Here's how the part is built. I have some questions about the finished solid (model axes, mm). A direction names the side the tool comes from. Coordinates: 2 decimals unless noted, no trailing zeros. Order: outer loops, then holes, each group sorted by start corner. A loop starts at its lowest first (then second) coordinate and runs counter-clockwise, first axis right, second up. Notation, with made-up numbers: (70, 28) -> (78, 28) arc R36 cw to (78, 63) -> close; hole circle Ø10 at (87.5, 17.5). An arc over 180 degrees is marked (long way). One line per item, written item: value. Start each with the question number.
```python
from build123d import *

# Parameters (mm, degrees)
SKETCH1_R           = 9.5
BOSS_EXTRUDE1_DEPTH = 1
SKETCH2_R           = 8.5
BOSS_EXTRUDE3_DEPTH = 4
SKETCH3_R           = 8.5
BOSS_EXTRUDE4_DEPTH = 4
CUT_EXTRUDE1_DEPTH  = 17.748134224


with BuildPart() as part:
    # Sketch1 → Boss-Extrude1 (new, symmetric)
    with BuildSketch(Plane.YZ):
        with Locations(Location((0, 0, 0), (0, 0, 270))):
            Circle(SKETCH1_R)
    extrude(amount=BOSS_EXTRUDE1_DEPTH, both=True)

    # Sketch2 → Boss-Extrude3 (add)
    with BuildSketch(Plane.YZ.offset(1)):
        with Locations(Location((-1, 0, 0), (0, 0, 180))):
            Circle(SKETCH2_R)
    extrude(amount=BOSS_EXTRUDE3_DEPTH)

    # Sketch3 → Boss-Extrude4 (add)
    with BuildSketch(Plane(origin=(-1, 0, 0), x_dir=(0, -1, 0), z_dir=(-1, 0, 0))):
        with Locations(Location((-1, 0, 0), (0, 0, 179.999143376))):
            Circle(SKETCH3_R)
    extrude(amount=BOSS_EXTRUDE4_DEPTH)

    # Sketch4 → Cut-Extrude1 (cut, through all)
    with BuildSketch(Plane.YZ.offset(5)):
        with BuildLine():
            Line((-1.5, 4.874423043), (-1.5, 6.7))
            Line((-1.5, 6.7), (1.5, 6.7))
            Line((1.5, 6.7), (1.5, 4.874423043))
            ThreePointArc((1.5, 4.874423043), (0, -5.1), (-1.5, 4.874423043))
        make_face()
    extrude(amount=-CUT_EXTRUDE1_DEPTH, mode=Mode.SUBTRACT)


solid = part.part
```
Q1. Imagine slicing it at A-A (x = 3). Write out the boundary of the cut face in (y, z), plus the area to 3 significant figures.
Q2. Imagine slicing it at D-D (z = -6.25). Write out the boundary of the cut face in (x, y).
Q3. Imagine slicing it at C-C (y = 0). Write out the boundary of the cut face in (x, z).
Q4. For P1, Ø2, axis at x = -2.5, y = 4.5, coming from the +Z side; P2, Ø0.5, axis at x = 2, z = 5.5, coming from the +Y side; P3, Ø1.5, axis at x = 2.5, z = 1.5, coming from the +Y side, each with a flat end and sliding along its axis, tell me the tip position at first contact or that it passes through.
Q5. For faces 4 (the face through (2.97, -9.11, -2.55)), 5 (the face through (-2.97, -0.84, 8.3)), 6 (the face through (0, 1.5, 6)), which set-ups out of +Z, -Z, +X, -X, +Y, -Y let a thin tool reach every point of the face, with its end or its side?
Q6. I need wall thicknesses on line 1 (Y direction, x = -1.25, z = 0); line 2 (Z direction, x = 0, y = 0); line 3 (Y direction, x = -0.5, z = 4). Which ranges of each line are inside material? Lowest first, please.
Q7. If we mould it in two halves opening along Z, with no side actions, what happens to faces 1 (the face through (0.01, -5.78, 7.54)), 2 (the face through (0, 0, 6.7)), 3 (the face through (5, -5, 4))? For each: +Z half, -Z half, draft (parallel to the pull), parting line (faces both ways), or undercut.
Completed:
1. outline: circle Ø17 at (-1, 0); hole (-1.5, 4.87) arc R5.1 ccw (long way) to (1.5, 4.87) -> (1.5, 6.7) -> (-1.5, 6.7) -> close
1. area: 140 mm2
2. outline: (-5, -4.76) -> (-1, -4.76) -> (-1, -7.15) -> (1, -7.15) -> (1, -6.76) -> (5, -6.76) -> (5, 4.76) -> (1, 4.76) -> (1, 7.15) -> (-1, 7.15) -> (-1, 6.76) -> (-5, 6.76) -> close
3. outline: (-5, -8.44) -> (-1, -8.44) -> (-1, -9.5) -> (1, -9.5) -> (1, -8.44) -> (5, -8.44) -> (5, -5.1) -> (-5, -5.1) -> close; (-5, 6.7) -> (5, 6.7) -> (5, 8.44) -> (1, 8.44) -> (1, 9.5) -> (-1, 9.5) -> (-1, 8.44) -> (-5, 8.44) -> close
4. P1: stops at z = 8.12
4. P2: stops at y = 5.68
4. P3: stops at y = 7.47
5. face 4: +X
5. face 5: -X
5. face 6: +X, -X
6. line 1: y = -7.5 to -5.1, 5.1 to 9.5
6. line 2: z = -9.5 to -5.1, 6.7 to 9.5
6. line 3: y = -8.62 to -3.16, 3.16 to 8.62
7. face 1: parting line
7. face 2: undercut
7. face 3: draft
